```python
from build123d import *

# Parameters (mm, degrees)
SKETCH1_W              = 150
SKETCH1_H              = 120
BOSS_EXTRUDE1_DEPTH    = 60
SKETCH2_W              = 10
SKETCH2_H              = 40
CUT_EXTRUDE1_DEPTH     = 60
CUT_EXTRUDE2_DEPTH     = 40
M20_TAPPED_HOLE1_D     = 17.5
M20_TAPPED_HOLE1_DEPTH = 67.5
M20_TAPPED_HOLE1_TIP   = 5.257530416
CUT_EXTRUDE4_DEPTH     = 30
M20_TAPPED_HOLE2_D     = 17.5
M20_TAPPED_HOLE2_DEPTH = 30
M20_TAPPED_HOLE2_TIP   = 5.257530416
M20_TAPPED_HOLE3_D     = 17.5
M20_TAPPED_HOLE3_DEPTH = 35
M20_TAPPED_HOLE3_TIP   = 5.257530416


with BuildPart() as part:
    # Sketch1 → Boss-Extrude1 (new body)
    with BuildSketch(Plane.XY):
        with Locations((75, 60)):
            Rectangle(SKETCH1_W, SKETCH1_H)
    extrude(amount=BOSS_EXTRUDE1_DEPTH)

    # Sketch2 → Cut-Extrude1 (cut)
    with BuildSketch(Plane.XY.offset(60)):
        with Locations((5, 90)):
            Rectangle(SKETCH2_W, SKETCH2_H)
        with Locations((5, 30)):
            Rectangle(SKETCH2_W, SKETCH2_H)
    extrude(amount=-CUT_EXTRUDE1_DEPTH, mode=Mode.SUBTRACT)

    # Sketch3 → Cut-Extrude2 (cut)
    with BuildSketch(Plane.XY.offset(60)):
        with BuildLine():
            Line((10, 110), (30, 110))
            ThreePointArc((30, 110), (50, 90), (30, 70))
            Line((30, 70), (10, 70))
            Line((10, 70), (10, 110))
        make_face()
        with BuildLine():
            Line((10, 50), (10, 10))
            Line((10, 10), (30, 10))
            ThreePointArc((30, 10), (50, 30), (30, 50))
            Line((30, 50), (10, 50))
        make_face()
    extrude(amount=-CUT_EXTRUDE2_DEPTH, mode=Mode.SUBTRACT)

    # M20 Tapped Hole1
    with Locations(Plane(origin=(30, 90, 20), x_dir=(1, 0, 0), z_dir=(0, 0, 1))):
        with Locations((0, 0), (0, -60)):
            Hole(M20_TAPPED_HOLE1_D / 2, depth=M20_TAPPED_HOLE1_DEPTH)
            with Locations((0, 0, -(M20_TAPPED_HOLE1_DEPTH + M20_TAPPED_HOLE1_TIP / 2))):  # 118° drill point
                Cone(0, M20_TAPPED_HOLE1_D / 2, M20_TAPPED_HOLE1_TIP, mode=Mode.SUBTRACT)

    # Sketch6 → Cut-Extrude4 (cut)
    with BuildSketch(Plane.XY.offset(60)):
        with BuildLine():
            ThreePointArc((30, 110), (35.176380902, 109.318516526), (40, 107.320508076))
            Line((40, 107.320508076), (40, 120))
            Line((40, 120), (0, 120))
            Line((0, 120), (0, 110))
            Line((0, 110), (30, 110))
        make_face()
        with BuildLine():
            Line((40, 47.320508076), (40, 72.679491924))
            ThreePointArc((40, 72.679491924), (35.176380902, 70.681483474), (30, 70))
            Line((30, 70), (0, 70))
            Line((0, 70), (0, 50))
            Line((0, 50), (30, 50))
            ThreePointArc((30, 50), (35.176380902, 49.318516526), (40, 47.320508076))
        make_face()
        with BuildLine():
            Line((40, 0), (40, 12.679491924))
            ThreePointArc((40, 12.679491924), (35.176380902, 10.681483474), (30, 10))
            Line((30, 10), (0, 10))
            Line((0, 10), (0, 0))
            Line((0, 0), (40, 0))
        make_face()
    extrude(amount=-CUT_EXTRUDE4_DEPTH, mode=Mode.SUBTRACT)

    # M20 Tapped Hole2
    with Locations(Plane(origin=(80, 60, 60), x_dir=(1, 0, 0), z_dir=(0, 0, 1))):
        with Locations((0, 0)):
            Hole(M20_TAPPED_HOLE2_D / 2, depth=M20_TAPPED_HOLE2_DEPTH)
            with Locations((0, 0, -(M20_TAPPED_HOLE2_DEPTH + M20_TAPPED_HOLE2_TIP / 2))):  # 118° drill point
                Cone(0, M20_TAPPED_HOLE2_D / 2, M20_TAPPED_HOLE2_TIP, mode=Mode.SUBTRACT)

    # M20 Tapped Hole3
    with Locations(Plane(origin=(150, 90, 40), x_dir=(0, 0, 1), z_dir=(1, 0, 0))):
        with Locations((0, 0), (0, 60)):
            Hole(M20_TAPPED_HOLE3_D / 2, depth=M20_TAPPED_HOLE3_DEPTH)
            with Locations((0, 0, -(M20_TAPPED_HOLE3_DEPTH + M20_TAPPED_HOLE3_TIP / 2))):  # 118° drill point
                Cone(0, M20_TAPPED_HOLE3_D / 2, M20_TAPPED_HOLE3_TIP, mode=Mode.SUBTRACT)


solid = part.part
```
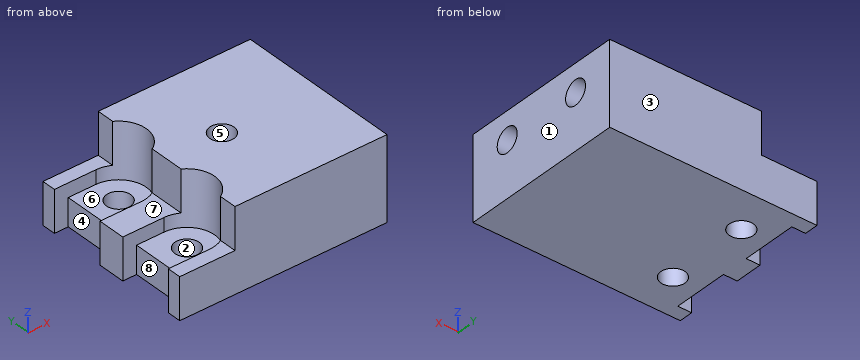
Geometry: final body of the model. Coordinates: model frame, mm. Face numbers are marked on the shaded views. A direction names the side the tool comes from. Coordinates: 2 decimals unless noted, no trailing zeros. Loops run counter-clockwise (first coordinate to the right, second up) from the corner with the lowest first, then second, coordinate; pieces in that order, holes last. Notation, with made-up numbers: M 84,77.5 L 137,77.5 A9 ccw 137,83.5 Z; hole C 15.5,-16 d7. An arc over 180 degrees is marked long. Put each result on its own line as item: value.
(1) Cut plane C-C on y = 16.5. Return the cut outline in (x, z), then the cut area to 3 significant figures.
Answer sheet:
outline: M 10,0 L 150,0 L 150,60 L 44.76,60 L 44.76,20 L 10,20 Z
area: 7,010 mm^2
(2) Access query for the marked faces 5, 6, 7 and 8. Directions: +Z, -Z, +X, -X, +Y, -Y. A direction counts if a zero-diameter tool reaches every point of the face in a straight line with its end or side. Return the directions, or none.
Answer sheet:
face 5: +Z
face 6: +Z, -X
face 7: +Z, -X, +Y, -Y
face 8: +Z, -Z, -X
(3) Cut plane A-A on z = 5. Return the cut outline in (x, y).
Answer sheet:
outline: M 0,0 L 150,0 L 150,120 L 0,120 L 0,110 L 10,110 L 10,70 L 0,70 L 0,50 L 10,50 L 10,10 L 0,10 Z; hole C 30,30 d17.5; hole C 30,90 d17.5
(4) First-contact query: pin 1 (4 mm diameter, centred on y = 5, z = 49, fed in from -X); pin 2 (16 mm diameter, centred on y = 100, z = 8.5, fed in from -X); pin 3 (20 mm diameter, centred on x = 36, y = 94, fed in from +Z). Flat tips, straight axial feed; report the tip coordinate or a pass-through.
Answer sheet:
pin 1: stops at x = 40
pin 2: stops at x = 10
pin 3: stops at z = 20
(5) Cut plane B-B on x = 28. Return the cut outline in (y, z), then the cut area to 3 significant figures.
Answer sheet:
outline: M 0,0 L 21.48,0 L 21.48,20 L 10,20 L 10,30 L 0,30 Z; M 38.52,0 L 81.48,0 L 81.48,20 L 70,20 L 70,30 L 50,30 L 50,20 L 38.52,20 Z; M 98.52,0 L 120,0 L 120,30 L 110,30 L 110,20 L 98.52,20 Z
area: 2,120 mm^2
(6) Draft query along X for the marked faces 1, 2, 3 and 4. Return one class per face: pulls with the +X half, pulls with the -X half, needs draft (parallel to the pull), parting line crosses it, or undercut.
Answer sheet:
face 1: pulls with the +X half
face 2: undercut
face 3: needs draft
face 4: pulls with the -X half
(7) Material intervals for probe 1 along Y at (x, z) = (138, 40); probe 2 along Y at (x, z) = (43, 38); probe 3 along Y at (x, z) = (80, 45), sorted ascending.
Answer sheet:
probe 1: y = 0 to 21.25, 38.75 to 81.25, 98.75 to 120
probe 2: y = 0 to 14.8, 45.2 to 74.8, 105.2 to 120
probe 3: y = 0 to 51.25, 68.75 to 120
